Geometry: final body of the model. Coordinates: model frame, mm. Give positions to 0.01 mm unless a question says otherwise; leave off trailing zeros. Loops run counter-clockwise (first coordinate to the right, second up) from the corner with the lowest first, then second, coordinate; pieces in that order, holes last. Notation, with made-up numbers: M -35,79 L 0,79 A15 ccw 0,95 Z; hole C -10,12 d8. An arc over 180 degrees is marked long. Put each result on its own line as item: value.
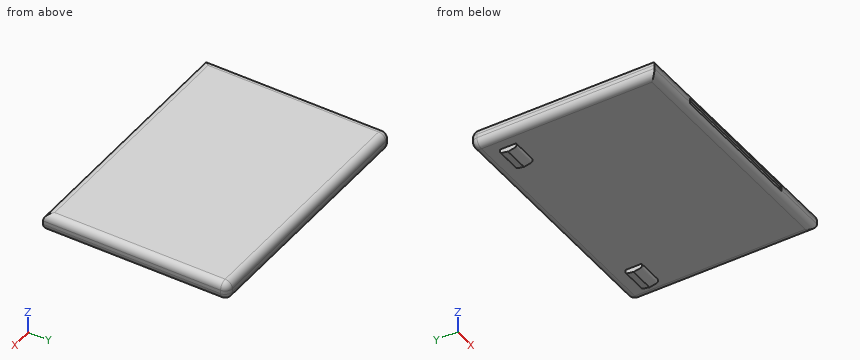
```python
from build123d import *

# Parameters (mm, degrees)
ESQUISSE1_W             = 356
ESQUISSE1_H             = 258.34
BOSS_EXTRU_1_DEPTH      = 25
CONG_1_R                = 10
BOSS_EXTRU_2_DEPTH      = 35
ESQUISSE4_W             = 200
ESQUISSE4_H             = 8
ENL_V_MAT_EXTRU_1_DEPTH = 3


with BuildPart() as part:
    # Esquisse1 → Boss.-Extru.1 (new body)
    with BuildSketch(Plane.XY):
        Rectangle(ESQUISSE1_W, ESQUISSE1_H)
    extrude(amount=BOSS_EXTRU_1_DEPTH)

    # Congé1
    cong_1_edges = [part.edges().sort_by_distance(p)[0] for p in [
        (178, 0, 25),
        (0, 129.17, 25),
        (-178, 0, 25),
        (0, 129.17, 0),
        (178, 0, 0),
        (0, -129.17, 0),
        (-178, 0, 0),
        (-178, 129.17, 12.5),
        (178, 129.17, 12.5),
        (0, -129.17, 25),
    ]]
    fillet(cong_1_edges, radius=CONG_1_R)

    # Esquisse3 → Boss.-Extru.2 (add)
    with BuildSketch(Plane(origin=(120, 0, 0), x_dir=(0, 0, -1), z_dir=(1, 0, 0))):
        with BuildLine():
            Line((0, 101.177924123), (0, 79.066125458))
            add(Edge.make_bspline(
                [(0, 79.066125458), (8.012390786, 75.823605097), (5.511301078, 85.583926919), (8.019330137, 90.12202479)],
                knots=[0, 0, 0, 0, 1, 1, 1, 1], degree=3))
            add(Edge.make_bspline(
                [(0, 101.177924123), (8.012390786, 104.420444484), (5.511301078, 94.660122661), (8.019330137, 90.12202479)],
                knots=[0, 0, 0, 0, 1, 1, 1, 1], degree=3))
        make_face()
    boss_extru_2 = extrude(amount=BOSS_EXTRU_2_DEPTH)

    # Symétrie1: Boss.-Extru.2 across plane
    add(boss_extru_2.mirror(Plane(origin=(0, 0, 0), x_dir=(0, 0, 1), z_dir=(1, 0, 0))))

    # Esquisse4 → Enlèv. mat.-Extru.1 (cut)
    with BuildSketch(Plane.XZ.offset(129.17)):
        with Locations((0, 12.5)):
            Rectangle(ESQUISSE4_W, ESQUISSE4_H)
    extrude(amount=-ENL_V_MAT_EXTRU_1_DEPTH, mode=Mode.SUBTRACT)


solid = part.part
```
Item 1: Line query: probe 1 along X at (y, z) = (97.5, -2); probe 2 along Z at (x, y) = (10, 85); probe 3 along Y at (x, z) = (-145.5, -2). Output: solid intervals per line, ascending. Write a range as [from, to].
Output values:
probe 1: [-155, -120], [120, 155]
probe 2: [0, 25]
probe 3: [78.48, 101.76]
Item 2: Section C-C on x = 37. Output: boundary loops of the cut face in (y, z).
Output values:
outline: M -129.06,8.5 A10 ccw -119.17,0 L 119.17,0 A10 ccw 129.17,10 L 129.17,15 A10 ccw 119.17,25 L -119.17,25 A10 ccw -129.06,16.5 L -126.17,16.5 L -126.17,8.5 Z
Item 3: Section A-A on x = -112.5. Output: boundary loops of the cut face in (y, z), then the cut area to 3 significant figures.
Output values:
outline: M -129.17,10 A10 ccw -119.17,0 L 119.17,0 A10 ccw 129.17,10 L 129.17,15 A10 ccw 119.17,25 L -119.17,25 A10 ccw -129.17,15 Z
area: 6,370 mm²
Item 4: Section B-B on y = 71.5. Output: boundary loops of the cut face in (x, z), then the cut area to 3 significant figures.
Output values:
outline: M -178,10 A10 ccw -168,0 L 168,0 A10 ccw 178,10 L 178,15 A10 ccw 168,25 L -168,25 A10 ccw -178,15 Z
area: 8,810 mm²
Item 5: Pin query (flat end, axial travel): pin 1 Ø2.5 at (x, y) = (-25.5, -128) entering from +Z; pin 2 Ø2.5 at (y, z) = (84.5, -5.5) entering from -X; pin 3 Ø8 at (x, y) = (25.5, -61.5) entering from -Z. Return the tip coordinate at first contact, or that it passes through.
Output values:
pin 1: z = 21.52
pin 2: x = -155
pin 3: z = 0
